from build123d import *

# Parameters (mm, degrees)
SKETCH1_W               = 25.4
SKETCH1_H               = 63.5
SKETCH1_H_2             = 12.7
BOSS_EXTRUDE1_DEPTH     = 160.782
CUT_EXTRUDE2_DEPTH      = 168.175421411
CUT_EXTRUDE2_DEPTH_BACK = 168.175421411
SKETCH5_R               = 3.175
CUT_EXTRUDE3_DEPTH      = 6.35
BOSS_EXTRUDE2_REACH     = 177.247
SKETCH1_5_W             = 25.4
SKETCH1_5_H             = 12.7
SKETCH8_W               = 25.4
SKETCH8_H               = 3.175
BOSS_EXTRUDE3_DEPTH     = 12.7
FILLET1_R               = 6.35


with BuildPart() as part:
    # Sketch1 → Boss-Extrude1 (new body)
    with BuildSketch(Plane(origin=(0, 0, 0), x_dir=(1, 0, 0), z_dir=(0, 1, 0))):
        with Locations((0, -6.35)):
            Rectangle(SKETCH1_W, SKETCH1_H)
        with Locations((0, 31.75)):
            Rectangle(SKETCH1_W, SKETCH1_H_2)
    extrude(amount=BOSS_EXTRUDE1_DEPTH)

    # Sketch4 → Cut-Extrude2 (cut, two sides: drawn at the far end of the back side and taken through both)
    with BuildSketch(Plane(origin=(12.7, 0, 0), x_dir=(0, 0, -1), z_dir=(1, 0, 0)).offset(-CUT_EXTRUDE2_DEPTH_BACK)):
        Polygon((38.1, 160.782), (-38.1, 160.782), (-38.1, 135.285836654), align=None)
    extrude(amount=CUT_EXTRUDE2_DEPTH + CUT_EXTRUDE2_DEPTH_BACK, mode=Mode.SUBTRACT)

    # Sketch5 → Cut-Extrude3 (cut)
    with BuildSketch(Plane(origin=(0, 133.129531097, 44.544517993), x_dir=(1, 0, 0), z_dir=(0, 0.9483236552061992, 0.3173046564050927))):
        with Locations(Location((0, 46.971851591, 0), (0, 0, 270))):
            Circle(SKETCH5_R)
    extrude(amount=-CUT_EXTRUDE3_DEPTH, mode=Mode.SUBTRACT)

    # Boss-Extrude2: from a plane face, 177.247 long prism both ways, kept between that surface and its translate by the depth
    boss_extrude2_start = Plane(origin=(-12.7, 135.285836654, 38.1), z_dir=(0, -0.9483236552061991, -0.31730465640509276)) * Box(710.988, 710.988, 355.494, align=(Align.CENTER, Align.CENTER, Align.MIN), mode=Mode.PRIVATE)
    boss_extrude2_end = Plane(origin=(-12.7, 144.810836654, 38.1), z_dir=(0, -0.9483236552061991, -0.31730465640509276)) * Box(710.988, 710.988, 355.494, align=(Align.CENTER, Align.CENTER, Align.MIN), mode=Mode.PRIVATE)
    # Sketch1_5 → Boss-Extrude2 (add, from a surface)
    with BuildSketch(Plane(origin=(0, 0, 0), x_dir=(1, 0, 0), z_dir=(0, 1, 0)), mode=Mode.PRIVATE) as boss_extrude2_sk1:
        with Locations((0, 31.75)):
            Rectangle(SKETCH1_5_W, SKETCH1_5_H)
    boss_extrude2_tool1 = extrude(boss_extrude2_sk1.sketch, amount=BOSS_EXTRUDE2_REACH, both=True, mode=Mode.PRIVATE)
    add(((boss_extrude2_tool1 - boss_extrude2_start) & boss_extrude2_end).solids().sort_by_distance((0, 161.295139, -31.75))[0])

    # Sketch8 → Boss-Extrude3 (add, along a direction that is not the sketch's normal)
    with BuildSketch(Plane.XY.offset(-25.4)):
        with Locations((0, 164.470139442)):
            Rectangle(SKETCH8_W, SKETCH8_H)
    extrude(amount=BOSS_EXTRUDE3_DEPTH, dir=(0, -0.31730465640509276, 0.9483236552061991))

    # Fillet1
    fillet1_edges = [part.edges().sort_by_distance(p)[0] for p in [
        (-12.7, 67.642918327, 38.1),
        (12.7, 67.642918327, 38.1),
        (-12.7, 85.1535, -38.1),
        (12.7, 85.1535, -38.1),
    ]]
    fillet(fillet1_edges, radius=FILLET1_R)


solid = part.part
Geometry check sheet. Reference: the model listing, model coordinates, mm. A direction names the side the tool comes from. Give positions to 0.01 mm unless a question says otherwise; leave off trailing zeros. Write each loop counter-clockwise with the first axis right and the second up, starting at its lowest first coordinate (ties: lowest second). Pieces come first, ordered by that corner, then holes.
1) Go/stop test with flat-tipped pins: pin 1 Ø4 at (x, z) = (-7.5, 15.5) entering from +Y; pin 2 Ø1 at (x, z) = (1.5, -24) entering from +Y; pin 3 Ø2.5 at (x, y) = (5, 160) entering from +Z. Record where each tip stops, or that it passes through.
Values follow:
pin 1: stops at y = 143.52
pin 2: stops at y = 165.76
pin 3: stops at z = -13.36
2) Cross-section at C-C (x = -9.5). Record the boundary of the cut face in (y, z), plus the area to 3 significant figures.
Values follow:
outline: (0, -37.26) - (170.03, -37.26) - (162.03, -13.36) - (158.85, -13.36) - (162.88, -25.4) - (156.53, -25.4) - (135.57, 37.26) - (0, 37.26) - close
area: 11,200 mm2
3) Cross-section at B-B (z = -15). Record the boundary of the cut face in (x, y).
Values follow:
outline: (-12.7, 0) - (12.7, 0) - (12.7, 153.05) - (-12.7, 153.05) - close; (-12.7, 159.4) - (12.7, 159.4) - (12.7, 162.58) - (-12.7, 162.58) - close
4) Thickness scan on line 1 (Y direction, x = 6.75, z = -14); line 2 (Z direction, x = 6.5, y = 113); line 3 (Y direction, x = 5, z = -19). Record the ranges inside material, lowest first.
Values follow:
line 1: y = 0 to 152.72, 159.07 to 162.24
line 2: z = -38.1 to 38.1
line 3: y = 0 to 154.39, 160.74 to 163.92
5) Set-up check for faces 4 (the face through (0.044, 142.026, -2.057)), 5 (the face through (-0.178, 160.896, -19.462)), 6 (the face through (-0.18, 145.76, 6.79)), 7 (the face through (0, 160, -13.356)): record each of +Z, -Z, +X, -X, +Y, -Y from which the full face is reachable in a straight line by a thin tool's end or side.
Values follow:
face 4: none
face 5: +X, -X
face 6: +Z, +X, -X
face 7: +Z, +X, -X, +Y
6) Cross-section at A-A (y = 54). Record the boundary of the cut face in (x, z), plus the area to 3 significant figures.
Values follow:
outline: (-12.7, -31.75) arc R6.35 ccw to (-6.35, -38.1) - (6.35, -38.1) arc R6.35 ccw to (12.7, -31.75) - (12.7, 31.75) arc R6.35 ccw to (6.35, 38.1) - (-6.35, 38.1) arc R6.35 ccw to (-12.7, 31.75) - close
area: 1,900 mm2
7) Release check for a two-part mould opening along Z. For faces 1 (the face through (-10.89, 69.67, 36.19)), 2 (the face through (0, 86, -38.1)), 3 (the face through (0, 160, -25.4)) record: released by +Z, released by -Z, zero draft, split by the parting line, or undercut.
Values follow:
face 1: released by +Z
face 2: released by -Z
face 3: undercut
8) Cross-section at D-D (z = -23.5). Record the boundary of the cut face in (x, y).
Values follow:
outline: (-12.7, 0) - (12.7, 0) - (12.7, 155.9) - (-12.7, 155.9) - close; (-12.7, 162.25) - (12.7, 162.25) - (12.7, 165.42) - (-12.7, 165.42) - close
